from build123d import *

# Parameters (mm, degrees)
BASE_FLANGE1_DEPTH = 100
SKETCH6_R          = 5.5
SKETCH6_R_2        = 2.75
CUT_EXTRUDE1_DEPTH = 10
SKETCH7_R          = 4
CUT_EXTRUDE2_DEPTH = 10


# Sheet-metal steps are written as plain solids
with BuildPart() as part:
    # Sketch1 → Base-Flange1 (new body)
    with BuildSketch(Plane.XY):
        with BuildLine():
            Line((0, 19.5), (0, 3.5))
            ThreePointArc((0, 3.5), (-1.025126266, 1.025126266), (-3.5, 0))
            Line((-3.5, 0), (-85, 0))
            Line((-85, 0), (-85, 1.5))
            Line((-85, 1.5), (-3.5, 1.5))
            ThreePointArc((-3.5, 1.5), (-2.085786438, 2.085786438), (-1.5, 3.5))
            Line((-1.5, 3.5), (-1.5, 19.5))
            Line((-1.5, 19.5), (0, 19.5))
        make_face()
    extrude(amount=BASE_FLANGE1_DEPTH)

    # Sketch6 → Cut-Extrude1 (cut)
    with BuildSketch(Plane.ZY.offset(1.5)):
        with Locations(Location((37, 10.5, 0), (0, 0, 270))):
            Circle(SKETCH6_R)
        with Locations(Location((8, 10.5, 0), (0, 0, 270))):
            Circle(SKETCH6_R_2)
        with Locations(Location((92, 10.5, 0), (0, 0, 90))):
            Circle(SKETCH6_R_2)
        with Locations(Location((63, 10.5, 0), (0, 0, 90))):
            Circle(SKETCH6_R)
    extrude(amount=-CUT_EXTRUDE1_DEPTH, mode=Mode.SUBTRACT)

    # Sketch7 → Cut-Extrude2 (cut)
    with BuildSketch(Plane(origin=(0, 1.5, 0), x_dir=(1, 0, 0), z_dir=(0, 1, 0))):
        with Locations(Location((-65.5, -50, 0), (0, 0, 180))):
            Circle(SKETCH7_R)
    extrude(amount=-CUT_EXTRUDE2_DEPTH, mode=Mode.SUBTRACT)


solid = part.part
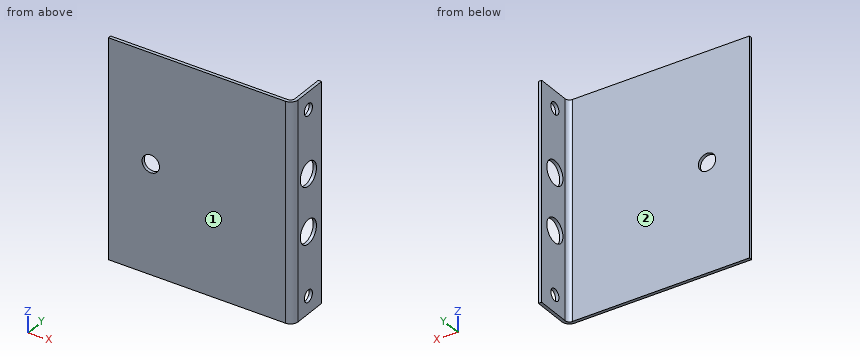
Check sheet for the modelled part. Datum: model origin and axes. Units: mm. Face numbers are marked on the shaded views. A direction names the side the tool comes from. Give positions to 0.01 mm unless a question says otherwise; leave off trailing zeros. Write each loop counter-clockwise with the first axis right and the second up, starting at its lowest first coordinate (ties: lowest second). Pieces come first, ordered by that corner, then holes. Notation, with made-up numbers: M -32.5,53.5 L 8.5,53.5 A19 cw 8.5,68.5 Z; hole C -34,26.25 d6. An arc over 180 degrees is marked long. Use one line per item in the form item = value.
(1) Section check C-C on y = 10.5. Record the boundary of the cut face in (x, z).
Answer block:
outline = M -1.5,0 L 0,0 L 0,5.25 L -1.5,5.25 Z; M -1.5,10.75 L 0,10.75 L 0,31.5 L -1.5,31.5 Z; M -1.5,42.5 L 0,42.5 L 0,57.5 L -1.5,57.5 Z; M -1.5,68.5 L 0,68.5 L 0,89.25 L -1.5,89.25 Z; M -1.5,94.75 L 0,94.75 L 0,100 L -1.5,100 Z
(2) Section check A-A on x = -65.5. Record the boundary of the cut face in (y, z).
Answer block:
outline = M 0,0 L 1.5,0 L 1.5,46 L 0,46 Z; M 0,54 L 1.5,54 L 1.5,100 L 0,100 Z
(3) Section check D-D on z = 72. Record the boundary of the cut face in (x, y).
Answer block:
outline = M -85,0 L -3.5,0 A3.5 ccw 0,3.5 L 0,19.5 L -1.5,19.5 L -1.5,3.5 A2 cw -3.5,1.5 L -85,1.5 Z
(4) Section check B-B on z = 37. Record the boundary of the cut face in (x, y).
Answer block:
outline = M -85,0 L -3.5,0 A3.5 ccw 0,3.5 L 0,5 L -1.5,5 L -1.5,3.5 A2 cw -3.5,1.5 L -85,1.5 Z; M -1.5,16 L 0,16 L 0,19.5 L -1.5,19.5 Z
(5) Depth check by flat-ended pin: P1, Ø1, axis at x = -34, y = 3, coming from the +Z side; P2, Ø6.5, axis at y = 10.5, z = 92, coming from the -X side; P3, Ø24.5, axis at x = -58, z = 26.5, coming from the +Y side. Enter the tip coordinate at first touch or a pass-through.
Answer block:
P1 = through
P2 = -1.5
P3 = 1.5
(6) Material ranges on line 1 along Z through (x, y) = (-0.85, 10.5); line 2 along Z through (x, y) = (-65.5, 0.95); line 3 along X through (y, z) = (4.5, 78), recorded low to high.
Answer block:
line_1 = 0 to 5.25, 10.75 to 31.5, 42.5 to 57.5, 68.5 to 89.25, 94.75 to 100
line_2 = 0 to 46, 54 to 100
line_3 = -1.5 to 0
(7) Tool access check on the marked faces 1 and 2. Record the directions out of +Z, -Z, +X, -X, +Y, -Y that give a thin tool (end or side, any length) a straight path to the whole face; none if there is none.
Answer block:
face_1 = +Z, -Z, +X, -X, -Y
face_2 = +Z, -Z, -X, +Y
